The drawing under review shows one solid part. Ordinate dimensions are in mm from its lowest x, y, z. Coordinates: 2 decimals unless noted, no trailing zeros. Loops run counter-clockwise (first coordinate to the right, second up) from the corner with the lowest first, then second, coordinate; pieces in that order, holes last. Notation, with made-up numbers: (87, 43.5) - (95, 43.5) arc R28 cw to (95, 68.5) - close; hole circle Ø8 at (69, 83.5). An arc over 180 degrees is marked (long way). Answer as a JSON object with one key per item and string values. Group by question number.
Item 1: We need section B-B (y = 3). Give the boundary of the cut face in (x, z).
Item 2: To check wall thickness, follow line 1 (Y direction, x = 3, z = 1.6); line 2 (X direction, y = 3.7, z = 2.75); line 3 (X direction, y = 2.8, z = 4.4). State the ranges of each line that lie inside material, in increasing order.
Item 3: Clearance check with a flat-ended pin moving along its axis: pin 1 (2 mm diameter, centred on x = 5, z = 1, fed in from -Y). State where the tip first meets the part, or that it passes through.
Item 4: We need section C-C (z = 0.45). Give the boundary of the cut face in (x, y).
Item 5: We need section A-A (x = 3). Give the boundary of the cut face in (y, z).
Item 6: Mouldability with a two-part tool opening along Y and no side actions: class the marked faces 1, 2 and 3 as released by +Y, released by -Y, zero draft, split by the parting line, or undercut.
Item 7: We need section D-D (x = 1.7). Give the boundary of the cut face in (y, z).
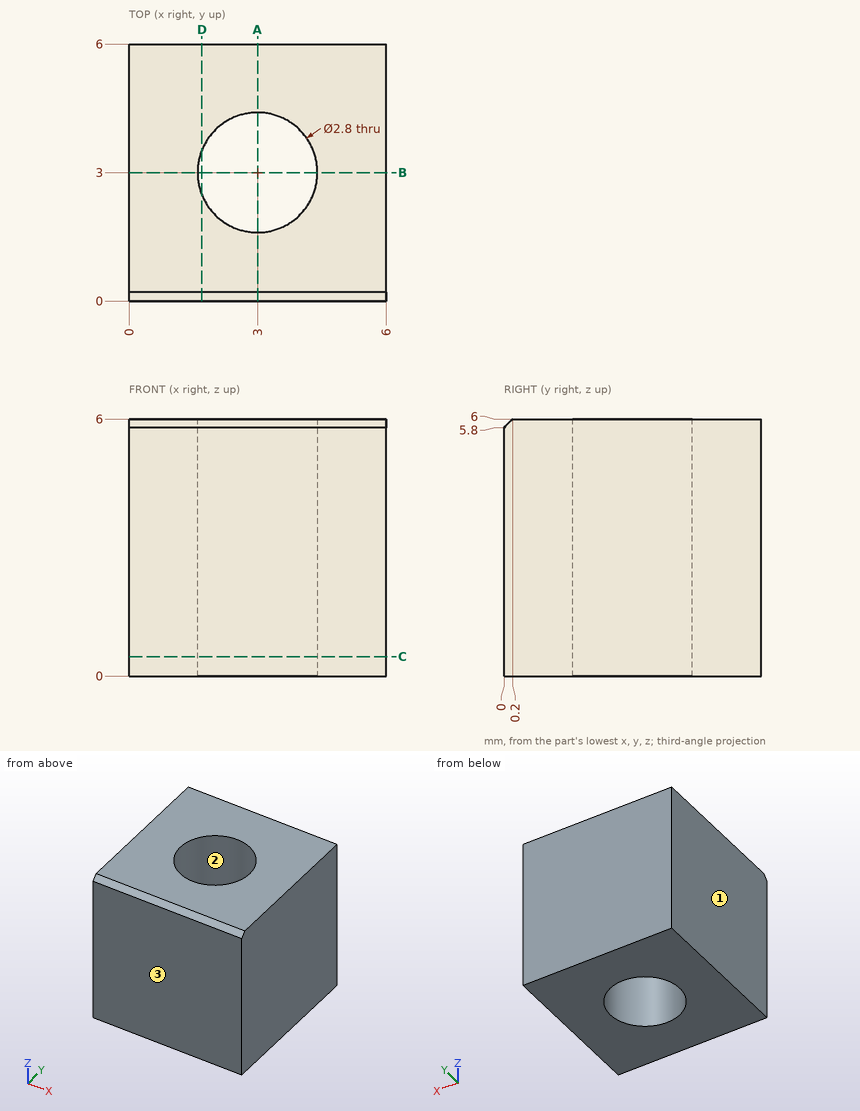
Check sheet entries:
{
 "1": {"outline": "(0, 0) - (1.6, 0) - (1.6, 6) - (0, 6) - close; (4.4, 0) - (6, 0) - (6, 6) - (4.4, 6) - close"},
 "2": {"line 1": "y = 0 to 1.6, 4.4 to 6", "line 2": "x = 0 to 1.79, 4.21 to 6", "line 3": "x = 0 to 1.61, 4.39 to 6"},
 "3": {"pin 1": "stops at y = 0"},
 "4": {"outline": "(0, 0) - (6, 0) - (6, 6) - (0, 6) - close; hole circle Ø2.8 at (3, 3)"},
 "5": {"outline": "(0, 0) - (1.6, 0) - (1.6, 6) - (0.2, 6) - (0, 5.8) - close; (4.4, 0) - (6, 0) - (6, 6) - (4.4, 6) - close"},
 "6": {"face 1": "zero draft", "face 2": "undercut", "face 3": "released by -Y"},
 "7": {"outline": "(0, 0) - (2.48, 0) - (2.48, 6) - (0.2, 6) - (0, 5.8) - close; (3.52, 0) - (6, 0) - (6, 6) - (3.52, 6) - close"}
}
